Here's how the part is built. I have some questions about the finished solid (model axes, mm). A direction names the side the tool comes from. Give positions to 0.01 mm unless a question says otherwise; leave off trailing zeros. Order: outer loops, then holes, each group sorted by start corner. A loop starts at its lowest first (then second) coordinate and runs counter-clockwise, first axis right, second up.
from build123d import *

# Parameters (mm, degrees)
SKETCH1_W               = 889
SKETCH1_H               = 127
BOSS_EXTRUDE1_DEPTH     = 177.8
SKETCH2_R               = 50.8
CUT_EXTRUDE1_DEPTH      = 496.3
SKETCH3_W               = 878.84
SKETCH3_H               = 116.84
SKETCH3_R               = 50.8
CUT_EXTRUDE2_DEPTH      = 2.54
SKETCH4_W               = 878.84
SKETCH4_H               = 116.84
CUT_EXTRUDE3_DEPTH      = 2.54
SKETCH5_W               = 177.8
SKETCH5_H               = 143.436769994
BOSS_EXTRUDE2_DEPTH     = 76.2
BOSS_EXTRUDE3_DEPTH     = 76.2
FILLET1_R               = 25.4
FILLET2_R               = 25.4
FILLET5_R               = 25.4
FILLET6_R               = 25.4
CUT_EXTRUDE5_DEPTH      = 25.4
CUT_EXTRUDE6_START      = -25.4
CUT_EXTRUDE6_DEPTH      = 25.4
CUT_EXTRUDE7_DEPTH      = 25.4
CUT_EXTRUDE7_DEPTH_BACK = 801.270015469
SKETCH12_W              = 279.4
SKETCH12_H              = 41.580374328
SKETCH12_H_2            = 85.419625672


with BuildPart() as part:
    # Sketch1 → Boss-Extrude1 (new body)
    with BuildSketch(Plane.XY):
        with Locations((0, -63.5)):
            Rectangle(SKETCH1_W, SKETCH1_H)
    extrude(amount=BOSS_EXTRUDE1_DEPTH)

    # Sketch2 → Cut-Extrude1 (cut, through all)
    with BuildSketch(Plane.XY.offset(177.8)):
        with Locations((0, -63.5)):
            Circle(SKETCH2_R)
    extrude(amount=-CUT_EXTRUDE1_DEPTH, mode=Mode.SUBTRACT)

    # Sketch3 → Cut-Extrude2 (cut)
    with BuildSketch(Plane.XY.offset(177.8)):
        with Locations((0, -63.5)):
            Rectangle(SKETCH3_W, SKETCH3_H)
        with Locations((0, -63.5)):
            Circle(SKETCH3_R, mode=Mode.SUBTRACT)
    extrude(amount=-CUT_EXTRUDE2_DEPTH, mode=Mode.SUBTRACT)

    # Sketch4 → Cut-Extrude3 (cut)
    with BuildSketch(Plane(origin=(0, 0, 0), x_dir=(-1, 0, 0), z_dir=(0, 0, -1))):
        with Locations((0, -63.5)):
            Rectangle(SKETCH4_W, SKETCH4_H)
    extrude(amount=-CUT_EXTRUDE3_DEPTH, mode=Mode.SUBTRACT)

    # Sketch5 → Boss-Extrude2 (add)
    with BuildSketch(Plane.ZY.offset(444.5)):
        Polygon((509.856034206, -575.236769994), (103.456034206, -575.236769994), (0, -270.436769994), (177.8, -270.436769994), (246.770689471, -473.636769994), (509.856034206, -493.059090132), align=None)
        with Locations((88.9, -198.718384997)):
            Rectangle(SKETCH5_W, SKETCH5_H)
    extrude(amount=-BOSS_EXTRUDE2_DEPTH)

    # Sketch8 → Boss-Extrude3 (add)
    with BuildSketch(Plane(origin=(444.5, 0, 0), x_dir=(0, 0, -1), z_dir=(1, 0, 0))):
        Polygon((-509.856034206, -575.236769994), (-103.456034206, -575.236769994), (0, -270.436769994), (0, -127), (-177.8, -127), (-177.8, -270.436769994), (-246.770689471, -473.636769994), (-509.856034206, -493.059090132), align=None)
    extrude(amount=-BOSS_EXTRUDE3_DEPTH)

    # Fillet1
    fillet1_edges = [part.edges().sort_by_distance(p)[0] for p in [
        (-406.4, -270.436769994, 177.8),
    ]]
    fillet(fillet1_edges, radius=FILLET1_R)

    # Fillet2
    fillet2_edges = [part.edges().sort_by_distance(p)[0] for p in [
        (406.4, -270.436769994, 177.8),
    ]]
    fillet(fillet2_edges, radius=FILLET2_R)

    # Fillet5
    fillet5_edges = [part.edges().sort_by_distance(p)[0] for p in [
        (444.5, -422.836769994, 51.728017103),
    ]]
    fillet(fillet5_edges, radius=FILLET5_R)

    # Fillet6
    fillet6_edges = [part.edges().sort_by_distance(p)[0] for p in [
        (-444.5, -422.836769994, 51.728017103),
    ]]
    fillet(fillet6_edges, radius=FILLET6_R)

    # Sketch10 → Cut-Extrude5 (cut)
    with BuildSketch(Plane(origin=(444.5, 0, 0), x_dir=(0, 0, -1), z_dir=(1, 0, 0))):
        with BuildLine():
            Line((-484.456034206, -549.836769994), (-148.481224008, -549.836769994))
            Line((-148.481224008, -549.836769994), (-25.4, -187.217447055))
            Line((-25.4, -187.217447055), (-25.4, -25.4))
            Line((-25.4, -25.4), (-152.4, -25.4))
            Line((-152.4, -25.4), (-152.4, -266.243582389))
            ThreePointArc((-152.4, -266.243582389), (-153.078401591, -274.517962908), (-155.095487125, -282.571345281))
            Line((-155.095487125, -282.571345281), (-228.125002086, -497.729371886))
            Line((-228.125002086, -497.729371886), (-484.456034206, -516.653053752))
            Line((-484.456034206, -516.653053752), (-484.456034206, -549.836769994))
        make_face()
    extrude(amount=-CUT_EXTRUDE5_DEPTH, mode=Mode.SUBTRACT)

    # Sketch11 → Cut-Extrude6 (cut)
    with BuildSketch(Plane.ZY.offset(444.5).offset(CUT_EXTRUDE6_START)):
        with BuildLine():
            Line((25.4, -25.4), (25.4, -187.217447055))
            Line((25.4, -187.217447055), (148.481224008, -549.836769994))
            Line((148.481224008, -549.836769994), (484.456034206, -549.836769994))
            Line((484.456034206, -549.836769994), (484.456034206, -516.653053752))
            Line((484.456034206, -516.653053752), (228.125002086, -497.729371886))
            Line((228.125002086, -497.729371886), (155.095487125, -282.571345281))
            ThreePointArc((155.095487125, -282.571345281), (153.078401591, -274.517962908), (152.4, -266.243582389))
            Line((152.4, -266.243582389), (152.4, -25.4))
            Line((152.4, -25.4), (25.4, -25.4))
        make_face()
    extrude(amount=CUT_EXTRUDE6_DEPTH, mode=Mode.SUBTRACT)

    # Sketch12 → Cut-Extrude7 (cut, two sides: drawn at the far end of the back side and taken through both)
    with BuildSketch(Plane.XY.offset(175.26).offset(-CUT_EXTRUDE7_DEPTH_BACK)):
        with Locations((-228.6, -101.129812836)):
            Rectangle(SKETCH12_W, SKETCH12_H)
        with Locations((-228.6, -164.629812836)):
            Rectangle(SKETCH12_W, SKETCH12_H_2)
        with Locations((228.6, -101.129812836)):
            Rectangle(SKETCH12_W, SKETCH12_H)
        with Locations((228.6, -164.629812836)):
            Rectangle(SKETCH12_W, SKETCH12_H_2)
    extrude(amount=CUT_EXTRUDE7_DEPTH + CUT_EXTRUDE7_DEPTH_BACK, mode=Mode.SUBTRACT)


solid = part.part
Q1. I'm going to push flat-ended pins straight in: P1, Ø12.5, axis at x = 435, y = -531.5, coming from the -Z side; P2, Ø20.5, axis at x = -429, z = 323, coming from the +Y side; P3, Ø20.5, axis at x = -435, y = -94, coming from the +Z side. Where does each tip first touch, or does it pass through?
Filled sheet:
P1: stops at z = 89.93
P2: stops at y = -478.51
P3: stops at z = 177.8
Q2. For faces 4 (the face through (432, -549.837, 319)), 5 (the face through (368.3, -386, 195)), 6 (the face through (-431.622, -391.656, 192.121)), which set-ups out of +Z, -Z, +X, -X, +Y, -Y let a thin tool reach every point of the face, with its end or its side?
Filled sheet:
face 4: +X
face 5: +Z, -Z, -Y
face 6: -X
Q3. If we section it at D-D on x = 385: List the corners of the cut face in (y, z) for me, plus the area to 3 significant figures.
Filled sheet:
outline: (-575.24, 103.46) - (-270.44, 0) - (-121.92, 0) - (-121.92, 2.54) - (-5.08, 2.54) - (-5.08, 0) - (0, 0) - (0, 177.8) - (-5.08, 177.8) - (-5.08, 175.26) - (-121.92, 175.26) - (-121.92, 177.8) - (-266.24, 177.8) arc R25.4 cw to (-274.41, 179.15) - (-473.64, 246.77) - (-493.06, 509.86) - (-575.24, 509.86) - close
area: 124,000 mm2
Q4. If we section it at B-B on y = -146: List the corners of the cut face in (x, z) for me.
Filled sheet:
outline: (-444.5, 0) - (-368.3, 0) - (-368.3, 177.8) - (-444.5, 177.8) - (-444.5, 152.4) - (-419.1, 152.4) - (-419.1, 25.4) - (-444.5, 25.4) - close; (368.3, 0) - (444.5, 0) - (444.5, 25.4) - (419.1, 25.4) - (419.1, 152.4) - (444.5, 152.4) - (444.5, 177.8) - (368.3, 177.8) - close
Q5. If we section it at C-C on y = -63.5: List the corners of the cut face in (x, z) for me, plus the area to 3 significant figures.
Filled sheet:
outline: (-444.5, 0) - (-439.42, 0) - (-439.42, 2.54) - (-50.8, 2.54) - (-50.8, 175.26) - (-439.42, 175.26) - (-439.42, 177.8) - (-444.5, 177.8) - (-444.5, 152.4) - (-419.1, 152.4) - (-419.1, 25.4) - (-444.5, 25.4) - close; (50.8, 2.54) - (439.42, 2.54) - (439.42, 0) - (444.5, 0) - (444.5, 25.4) - (419.1, 25.4) - (419.1, 152.4) - (444.5, 152.4) - (444.5, 177.8) - (439.42, 177.8) - (439.42, 175.26) - (50.8, 175.26) - close
area: 130,000 mm2
Q6. Thinking about a two-plate mould opening in X: for faces 1 (the face through (437.257, -428.993, 61.884)), 2 (the face through (88.9, -103, 88)), 3 (the face through (-406.933, -372.628, 212.486)), which applies, released by +X, released by -X, zero draft, split by the parting line, or undercut?
Filled sheet:
face 1: released by +X
face 2: undercut
face 3: zero draft
Q7. I need wall thicknesses on L1, parallel to X at y = -118.5, z = 173.5; L2, parallel to X at y = -128, z = 67; L3, parallel to Y at x = 0, z = 54. Which ranges of each line are inside material? Lowest first, please.
Filled sheet:
L1: x = -444.5 to -368.3, -88.9 to 88.9, 368.3 to 444.5
L2: x = -419.1 to -368.3, 368.3 to 419.1
L3: y = -127 to -114.3, -12.7 to 0
Q8. If we section it at A-A on x = 0: List the corners of the cut face in (y, z) for me, plus the area to 3 significant figures.
Filled sheet:
outline: (-127, 0) - (-121.92, 0) - (-121.92, 2.54) - (-114.3, 2.54) - (-114.3, 175.26) - (-121.92, 175.26) - (-121.92, 177.8) - (-127, 177.8) - close; (-12.7, 2.54) - (-5.08, 2.54) - (-5.08, 0) - (0, 0) - (0, 177.8) - (-5.08, 177.8) - (-5.08, 175.26) - (-12.7, 175.26) - close
area: 4,440 mm2
